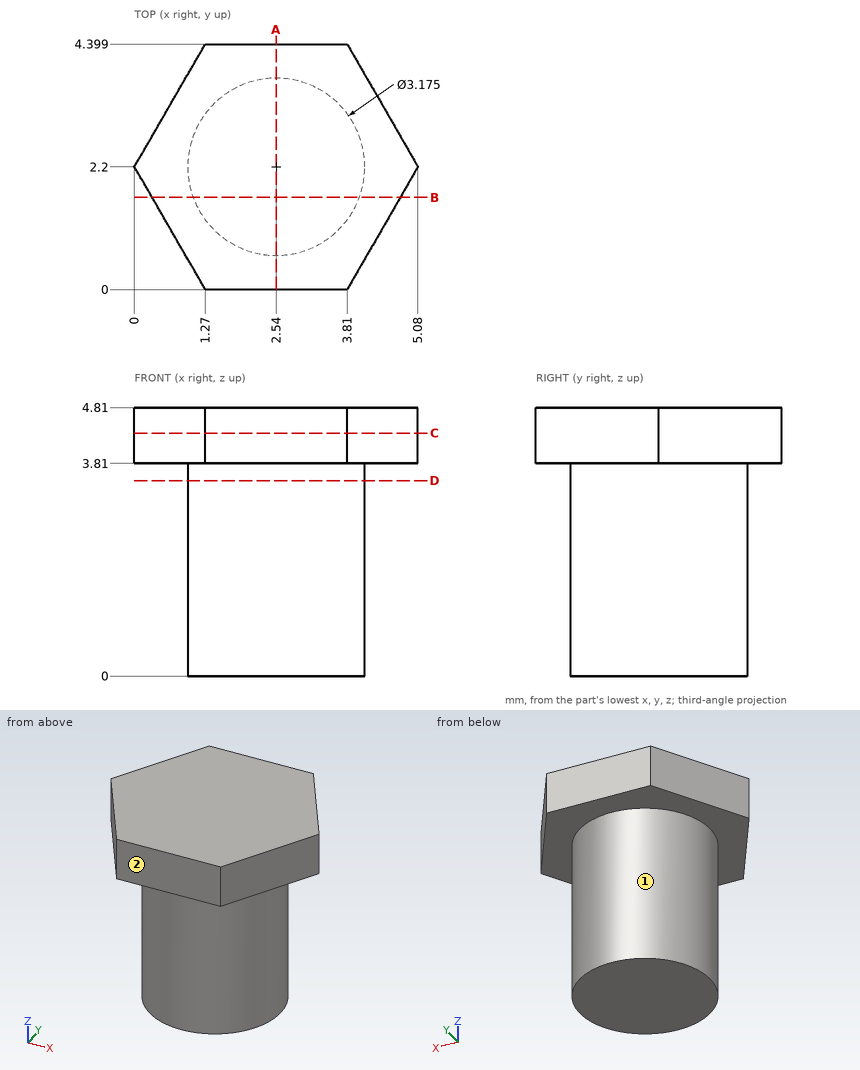
The figure shows three views and two pictorial views of one solid part (mm, origin at its lowest corner). Answer the questions. A direction names the side the tool comes from. Give positions to 0.01 mm unless a question says otherwise; leave off trailing zeros. Loops run counter-clockwise (first coordinate to the right, second up) from the corner with the lowest first, then second, coordinate; pieces in that order, holes last. Notation, with made-up numbers: (67.5, 39) - (87.5, 39) arc R31 cw to (87.5, 74) - close; hole circle Ø10 at (-29.75, 38.5). An arc over 180 degrees is marked (long way). Answer in a Markdown table with one row per item.
(1) Section B-B (y = 1.65) is taken. Give the vertices of the cut face in (x, z).
Results list:
| item | result |
|---|---|
| outline | (0.32, 3.81) - (1.05, 3.81) - (1.05, 0) - (4.03, 0) - (4.03, 3.81) - (4.76, 3.81) - (4.76, 4.81) - (0.32, 4.81) - close |
(2) Consider L1, parallel to Z at x = 1.9, y = 3.7; L2, parallel to Y at x = 3.25, z = 2.65; L3, parallel to Y at x = 3.7, z = 3.35 (1 decimal). Determine where each line is inside the solid, lowest interval first. Write a range as [from, to].
Results list:
| item | result |
|---|---|
| L1 | z = [3.81, 4.81] |
| L2 | y = [0.78, 3.62] |
| L3 | y = [1.1, 3.3] |
(3) Section A-A (x = 2.54) is taken. Give the vertices of the cut face in (y, z), and give its area (3 significant figures).
Results list:
| item | result |
|---|---|
| outline | (0, 3.81) - (0.61, 3.81) - (0.61, 0) - (3.79, 0) - (3.79, 3.81) - (4.4, 3.81) - (4.4, 4.81) - (0, 4.81) - close |
| area | 16.5 mm² |
(4) Section C-C (z = 4.35) is taken. Give the vertices of the cut face in (x, y).
Results list:
| item | result |
|---|---|
| outline | (0, 2.2) - (1.27, 0) - (3.81, 0) - (5.08, 2.2) - (3.81, 4.4) - (1.27, 4.4) - close |
(5) A tool of negligible diameter and unlimited length cuts with its end or side. For the marked faces 1 and 2, from which of +Z, -Z, +X, -X, +Y, -Y can it reach the whole face along a straight path? Write none if from no direction.
Results list:
| item | result |
|---|---|
| face 1 | -Z |
| face 2 | +Z, -Z, +X, -X, -Y |
(6) Flat-ended cylindrical pins translate along their axes: pin 1 Ø1.5 at (y, z) = (2.5, 1) entering from -X; pin 2 Ø1.5 at (x, z) = (2.5, 2) entering from -Y. Find the tip coordinate at first contact, or state that the pin passes through.
Results list:
| item | result |
|---|---|
| pin 1 | stops at x = 0.95 |
| pin 2 | stops at y = 0.61 |
(7) Section D-D (z = 3.5) is taken. Give the vertices of the cut face in (x, y) (1 decimal).
Results list:
| item | result |
|---|---|
| outline | circle Ø3.2 at (2.5, 2.2) |
